```python
from build123d import *

# Parameters (mm, degrees)
F0_W     = 60
F0_H     = 20
F0_W_2   = 34
F0_H_2   = 15
F1_DEPTH = 18


with BuildPart() as f1:
    # F0 (on Top) → F1 (new body)
    with BuildSketch(Plane.XY):
        with BuildLine():
            ThreePointArc((115.136532, 510.208606), (95.852904, 503.18994), (85.592299, 485.418052))
            Line((85.592299, 485.418052), (6.208375, 35.209445))
            ThreePointArc((6.208375, 35.209445), (12.771274, 10.716372), (35.752608, 0))
            Line((35.752608, 0), (296.236987, 0))
            ThreePointArc((296.236987, 0), (302.664863, 2.339556), (306.085065, 8.263518))
            Line((306.085065, 8.263518), (313.444333, 50))
            Line((313.444333, 50), (352.236268, 270))
            Line((352.236268, 270), (390.899802, 489.271795))
            Line((390.899802, 489.271795), (390.899802, 500.208606))
            ThreePointArc((390.899802, 500.208606), (387.97087, 507.279674), (380.899802, 510.208606))
            Line((380.899802, 510.208606), (115.136532, 510.208606))
        make_face()
        with Locations((69.279147, 40)):
            Rectangle(F0_W, F0_H, mode=Mode.SUBTRACT)
        with Locations((209.279147, 40)):
            Rectangle(F0_W, F0_H, mode=Mode.SUBTRACT)
        Polygon((303.92738, 63.435029), (290.492351, 50), (279.885749, 39.393398), (269.279147, 50), (293.320778, 74.041631), align=None, mode=Mode.SUBTRACT)
        with Locations((108.071083, 260)):
            Rectangle(F0_W, F0_H, mode=Mode.SUBTRACT)
        with Locations((146.899802, 480.208606)):
            Rectangle(F0_W, F0_H, mode=Mode.SUBTRACT)
        with Locations((248.071083, 260)):
            Rectangle(F0_W, F0_H, mode=Mode.SUBTRACT)
        Polygon((342.719315, 283.435029), (329.284287, 270), (318.677685, 259.393398), (308.071083, 270), (332.112714, 294.041631), align=None, mode=Mode.SUBTRACT)
        with Locations((213.899802, 482.708606)):
            Rectangle(F0_W_2, F0_H_2, mode=Mode.SUBTRACT)
        with Locations((281.899802, 480.208606)):
            Rectangle(F0_W, F0_H, mode=Mode.SUBTRACT)
        with Locations((353.899802, 482.708606)):
            Rectangle(F0_W_2, F0_H_2, mode=Mode.SUBTRACT)
    extrude(amount=F1_DEPTH)


solid = f1.part
```
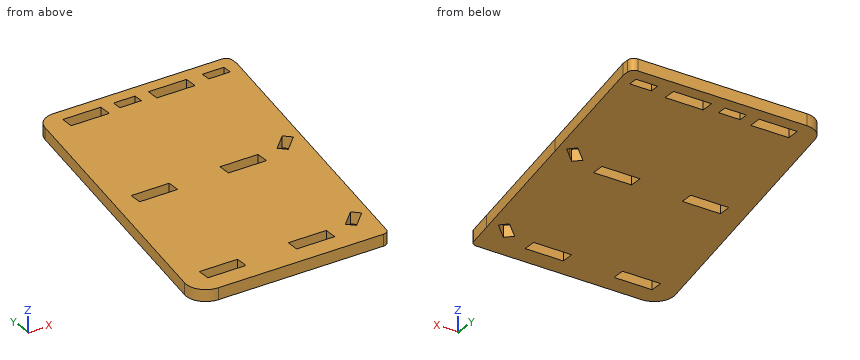
Model file for the job. Use its own axes, mm. Give positions to 0.01 mm unless a question says otherwise; leave off trailing zeros. Write each loop counter-clockwise with the first axis right and the second up, starting at its lowest first coordinate (ties: lowest second). Pieces come first, ordered by that corner, then holes. Notation, with made-up numbers: (50, 17) -> (97, 17) arc R15 cw to (97, 30) -> close; hole circle Ø5 at (78, -26). An arc over 180 degrees is marked (long way). Use CSV: the item, a comma, the result in double quotes. Start each with the question number.
1) Drill centre lines: L1, parallel to Y at x = 216, z = 14.5; L2, parallel to Y at x = 150.5, z = 17.25; L3, parallel to Y at x = 89, z = 2.5. Where is each one in solid material? Low to high.
2) Cut at A-A on x = 156. List the corners of the cut face in (y, z), plus the area to 3 significant figures.
3) Cut at B-B on z = 6.25. Count the separate pieces of the cut face and the enclosed holes in it, plus the area to 3 significant figures.
4) Pin check, flat tips, straight feed: P1, Ø4, axis at y = 107, z = 8.5, coming from the +X side; P2, Ø5.5, axis at y = 40.5, z = 12, coming from the -X side; P3, Ø6, axis at y = 168, z = 3.5, coming from the -X side; P4, Ø1.5, axis at x = 65, y = 382, coming from the -Z side. Stop position of each tip, or through.
5) Cut at D-D on y = 165.5. List the corners of the cut face in (x, z).
6) Cut at C-C on x = 105. List the corners of the cut face in (y, z).
Final values:
1,L1,"y = 0 to 30, 50 to 475.21, 490.21 to 510.21"
1,L2,"y = 0 to 470.21, 490.21 to 510.21"
1,L3,"y = 0 to 30, 50 to 250, 270 to 494.94"
2,outline,"(0, 0) -> (470.21, 0) -> (470.21, 18) -> (0, 18) -> close; (490.21, 0) -> (510.21, 0) -> (510.21, 18) -> (490.21, 18) -> close"
2,area,"8,820 mm2"
3,separate pieces,"1"
3,enclosed holes,"10"
3,area,"146,000 mm2"
4,P1,"stops at x = 323.85"
4,P2,"stops at x = 6.66"
4,P3,"stops at x = 29.09"
4,P4,"passes through"
5,outline,"(29.18, 0) -> (333.81, 0) -> (333.81, 18) -> (29.18, 18) -> close"
6,outline,"(0, 0) -> (250, 0) -> (250, 18) -> (0, 18) -> close; (270, 0) -> (508.44, 0) -> (508.44, 18) -> (270, 18) -> close"
